from build123d import *

# Parameters (mm, degrees)
BOSS_EXTRUDE1_DEPTH = 140
SKETCH1_5_R         = 0.75
BOSS_EXTRUDE2_DEPTH = 5
SKETCH2_R           = 0.9
SKETCH2_R_2         = 0.75
CUT_EXTRUDE1_DEPTH  = 6
SKETCH3_W           = 0.25
SKETCH3_H           = 2.7
CUT_EXTRUDE2_DEPTH  = 171.537268104
SKETCH4_W           = 13
SKETCH4_H           = 1.35
SKETCH4_W_2         = 24
SKETCH4_W_3         = 6
SKETCH4_W_4         = 7
SKETCH4_W_5         = 30
SKETCH4_W_6         = 4
CUT_EXTRUDE4_DEPTH  = 86.663575277
SKETCH6_W           = 13
SKETCH6_H           = 1.35
SKETCH6_W_2         = 24
SKETCH6_W_3         = 6
SKETCH6_W_4         = 7
SKETCH6_W_5         = 4
SKETCH6_W_6         = 20
CUT_EXTRUDE5_DEPTH  = 86.765556194
SKETCH7_W           = 20
SKETCH7_H           = 1.8
CUT_EXTRUDE6_DEPTH  = 86.663575277
SKETCH8_W           = 20
SKETCH8_H           = 1.8
CUT_EXTRUDE7_DEPTH  = 86.765556194


with BuildPart() as part:
    # Sketch1 → Boss-Extrude1 (new body)
    with BuildSketch(Plane(origin=(-58.146340827, 0, 0), x_dir=(0, 0, -1), z_dir=(1, 0, 0))):
        Polygon((-20.52887033, 84.640306989), (-21.87887033, 84.640306989), (-21.87887033, 85.940306989), (-21.37887033, 85.940306989), (-21.37887033, 86.490306989), (-23.17887033, 86.490306989), (-23.17887033, 85.940306989), (-22.67887033, 85.940306989), (-22.67887033, 84.640306989), (-24.02887033, 84.640306989), (-24.02887033, 76.840306989), (-13.52887033, 76.840306989), (-13.52887033, 77.640306989), (-14.87887033, 77.640306989), (-14.87887033, 78.940306989), (-14.37887033, 78.940306989), (-14.37887033, 79.490306989), (-16.17887033, 79.490306989), (-16.17887033, 78.940306989), (-15.67887033, 78.940306989), (-15.67887033, 77.640306989), (-17.02887033, 77.640306989), (-17.02887033, 80.340306989), (-20.52887033, 80.340306989), align=None)
    extrude(amount=BOSS_EXTRUDE1_DEPTH)

    # Sketch1_5 → Boss-Extrude2 (add)
    with BuildSketch(Plane(origin=(-58.146340827, 0, 0), x_dir=(0, 0, -1), z_dir=(1, 0, 0))):
        with Locations((-22.27887033, 82.090306989)):
            Circle(SKETCH1_5_R)
        with Locations((-18.77887033, 78.590306989)):
            Circle(SKETCH1_5_R)
    extrude(amount=-BOSS_EXTRUDE2_DEPTH)

    # Sketch2 → Cut-Extrude1 (cut)
    with BuildSketch(Plane(origin=(81.853659173, 0, 0), x_dir=(0, 0, -1), z_dir=(1, 0, 0))):
        with Locations((-22.27887033, 82.090306989)):
            Circle(SKETCH2_R)
        with Locations((-22.27887033, 82.090306989)):
            Circle(SKETCH2_R_2, mode=Mode.SUBTRACT)
        with Locations((-22.27887033, 82.090306989)):
            Circle(SKETCH2_R_2)
        with Locations((-18.77887033, 78.590306989)):
            Circle(SKETCH2_R)
        with Locations((-18.77887033, 78.590306989)):
            Circle(SKETCH2_R_2, mode=Mode.SUBTRACT)
        with Locations((-18.77887033, 78.590306989)):
            Circle(SKETCH2_R_2)
    extrude(amount=-CUT_EXTRUDE1_DEPTH, mode=Mode.SUBTRACT)

    # Sketch3 → Cut-Extrude2 (cut, through all)
    with BuildSketch(Plane(origin=(81.853659173, 0, 0), x_dir=(0, 0, -1), z_dir=(1, 0, 0))):
        with Locations((-17.15387033, 78.990306989)):
            Rectangle(SKETCH3_W, SKETCH3_H)
    extrude(amount=-CUT_EXTRUDE2_DEPTH, mode=Mode.SUBTRACT)

    # Sketch4 → Cut-Extrude4 (cut, through all)
    with BuildSketch(Plane(origin=(0, 84.640306989, 0), x_dir=(1, 0, 0), z_dir=(0, 1, 0))):
        with Locations((75.353659173, -23.35387033)):
            Rectangle(SKETCH4_W, SKETCH4_H)
        with Locations((53.853659173, -21.20387033)):
            Rectangle(SKETCH4_W_2, SKETCH4_H)
        with Locations((53.853659173, -23.35387033)):
            Rectangle(SKETCH4_W_2, SKETCH4_H)
        with Locations((38.853659173, -21.20387033)):
            Rectangle(SKETCH4_W_3, SKETCH4_H)
        with Locations((38.853659173, -23.35387033)):
            Rectangle(SKETCH4_W_3, SKETCH4_H)
        with Locations((32.353659173, -21.20387033)):
            Rectangle(SKETCH4_W_4, SKETCH4_H)
        with Locations((32.353659173, -23.35387033)):
            Rectangle(SKETCH4_W_4, SKETCH4_H)
        with Locations((13.853659173, -23.35387033)):
            Rectangle(SKETCH4_W_2, SKETCH4_H)
        with Locations((13.853659173, -21.20387033)):
            Rectangle(SKETCH4_W_2, SKETCH4_H)
        with Locations((-1.146340827, -21.20387033)):
            Rectangle(SKETCH4_W_3, SKETCH4_H)
        with Locations((-1.146340827, -23.35387033)):
            Rectangle(SKETCH4_W_3, SKETCH4_H)
        with Locations((-7.646340827, -21.20387033)):
            Rectangle(SKETCH4_W_4, SKETCH4_H)
        with Locations((-7.646340827, -23.35387033)):
            Rectangle(SKETCH4_W_4, SKETCH4_H)
        with Locations((-26.146340827, -21.20387033)):
            Rectangle(SKETCH4_W_2, SKETCH4_H)
        with Locations((-26.146340827, -23.35387033)):
            Rectangle(SKETCH4_W_2, SKETCH4_H)
        with Locations((-41.146340827, -23.35387033)):
            Rectangle(SKETCH4_W_3, SKETCH4_H)
        with Locations((-41.146340827, -21.20387033)):
            Rectangle(SKETCH4_W_3, SKETCH4_H)
        with Locations((-47.646340827, -21.20387033)):
            Rectangle(SKETCH4_W_4, SKETCH4_H)
        with Locations((-47.646340827, -23.35387033)):
            Rectangle(SKETCH4_W_4, SKETCH4_H)
        with Locations((-69.146340827, -21.20387033)):
            Rectangle(SKETCH4_W_5, SKETCH4_H)
        with Locations((-56.146340827, -23.35387033)):
            Rectangle(SKETCH4_W_6, SKETCH4_H)
        with Locations((75.353659173, -21.20387033)):
            Rectangle(SKETCH4_W, SKETCH4_H)
    extrude(amount=CUT_EXTRUDE4_DEPTH, mode=Mode.SUBTRACT)

    # Sketch6 → Cut-Extrude5 (cut, through all)
    with BuildSketch(Plane(origin=(0, 77.640306989, 0), x_dir=(1, 0, 0), z_dir=(0, 1, 0))):
        with Locations((75.353659173, -16.35387033)):
            Rectangle(SKETCH6_W, SKETCH6_H)
        with Locations((75.353659173, -14.20387033)):
            Rectangle(SKETCH6_W, SKETCH6_H)
        with Locations((53.853659173, -14.20387033)):
            Rectangle(SKETCH6_W_2, SKETCH6_H)
        with Locations((53.853659173, -16.35387033)):
            Rectangle(SKETCH6_W_2, SKETCH6_H)
        with Locations((38.853659173, -14.20387033)):
            Rectangle(SKETCH6_W_3, SKETCH6_H)
        with Locations((38.853659173, -16.35387033)):
            Rectangle(SKETCH6_W_3, SKETCH6_H)
        with Locations((32.353659173, -16.35387033)):
            Rectangle(SKETCH6_W_4, SKETCH6_H)
        with Locations((32.353659173, -14.20387033)):
            Rectangle(SKETCH6_W_4, SKETCH6_H)
        with Locations((13.853659173, -16.35387033)):
            Rectangle(SKETCH6_W_2, SKETCH6_H)
        with Locations((13.853659173, -14.20387033)):
            Rectangle(SKETCH6_W_2, SKETCH6_H)
        with Locations((-1.146340827, -16.35387033)):
            Rectangle(SKETCH6_W_3, SKETCH6_H)
        with Locations((-1.146340827, -14.20387033)):
            Rectangle(SKETCH6_W_3, SKETCH6_H)
        with Locations((-7.646340827, -14.20387033)):
            Rectangle(SKETCH6_W_4, SKETCH6_H)
        with Locations((-7.646340827, -16.35387033)):
            Rectangle(SKETCH6_W_4, SKETCH6_H)
        with Locations((-26.146340827, -14.20387033)):
            Rectangle(SKETCH6_W_2, SKETCH6_H)
        with Locations((-26.146340827, -16.35387033)):
            Rectangle(SKETCH6_W_2, SKETCH6_H)
        with Locations((-41.146340827, -14.20387033)):
            Rectangle(SKETCH6_W_3, SKETCH6_H)
        with Locations((-41.146340827, -16.35387033)):
            Rectangle(SKETCH6_W_3, SKETCH6_H)
        with Locations((-47.646340827, -16.35387033)):
            Rectangle(SKETCH6_W_4, SKETCH6_H)
        with Locations((-47.646340827, -14.20387033)):
            Rectangle(SKETCH6_W_4, SKETCH6_H)
        with Locations((-56.146340827, -14.20387033)):
            Rectangle(SKETCH6_W_5, SKETCH6_H)
        with Locations((-66.146340827, -16.35387033)):
            Rectangle(SKETCH6_W_2, SKETCH6_H)
        with Locations((-68.146340827, -14.20387033)):
            Rectangle(SKETCH6_W_6, SKETCH6_H)
    extrude(amount=CUT_EXTRUDE5_DEPTH, mode=Mode.SUBTRACT)

    # Sketch7 → Cut-Extrude6 (cut, through all)
    with BuildSketch(Plane(origin=(0, 84.640306989, 0), x_dir=(1, 0, 0), z_dir=(0, 1, 0))):
        with Locations((55.853659173, -22.27887033)):
            Rectangle(SKETCH7_W, SKETCH7_H)
        with Locations((15.853659173, -22.27887033)):
            Rectangle(SKETCH7_W, SKETCH7_H)
        with Locations((-24.146340827, -22.27887033)):
            Rectangle(SKETCH7_W, SKETCH7_H)
        with Locations((-64.146340827, -22.27887033)):
            Rectangle(SKETCH7_W, SKETCH7_H)
    extrude(amount=CUT_EXTRUDE6_DEPTH, mode=Mode.SUBTRACT)

    # Sketch8 → Cut-Extrude7 (cut, through all)
    with BuildSketch(Plane(origin=(0, 77.640306989, 0), x_dir=(1, 0, 0), z_dir=(0, 1, 0))):
        with Locations((55.853659173, -15.27887033)):
            Rectangle(SKETCH8_W, SKETCH8_H)
        with Locations((15.853659173, -15.27887033)):
            Rectangle(SKETCH8_W, SKETCH8_H)
        with Locations((-24.146340827, -15.27887033)):
            Rectangle(SKETCH8_W, SKETCH8_H)
        with Locations((-64.146340827, -15.27887033)):
            Rectangle(SKETCH8_W, SKETCH8_H)
    extrude(amount=CUT_EXTRUDE7_DEPTH, mode=Mode.SUBTRACT)


solid = part.part
Input: part model. Units: mm. Frame: model coordinates. A direction names the side the tool comes from. Coordinates: 2 decimals unless noted, no trailing zeros. Loops run counter-clockwise (first coordinate to the right, second up) from the corner with the lowest first, then second, coordinate; pieces in that order, holes last.
(1) Pull-direction query (Z, two-part tool) for faces 4 (the face through (11, 76.84, 19)), 5 (the face through (11, 82, 20.529)), 6 (the face through (13, 77.64, 15)); classes: released by +Z, released by -Z, zero draft, split by the parting line, or undercut.
(2) Material intervals for probe 1 along Z at (x, y) = (-47, 79.25); probe 2 along Y at (x, z) = (-55, 18.75); probe 3 along X at (y, z) = (83, 21.25), sorted ascending.
(3) Section B-B on x = 32. Return the cut outline in (y, z), then the cut area to 3 significant figures.
(4) Set-up query: faces 1 (the face through (11, 81, 24.029)), 2 (the face through (11, 80.34, 19)), 3 (the face through (13, 79, 17.279)). Return all of +Z, -Z, +X, -X, +Y, -Y with unobstructed straight access to the full face (end or side cutting, diameter ignored); none if empty.
(5) Section A-A on x = -26. Return the cut outline in (y, z).
(6) First-contact query: pin 1 Ø0.6 at (x, y) = (27, 86.5) entering from -Z; pin 2 Ø0.6 at (x, y) = (-53.5, 79) entering from -Z; pin 3 Ø1.5 at (x, y) = (37.5, 86) entering from -Z. Flat tips, straight axial feed; report the tip coordinate or a pass-through.
Data:
1. face 4: zero draft
1. face 5: released by -Z
1. face 6: undercut
2. probe 1: z = 14.88 to 15.68, 17.28 to 24.03
2. probe 2: y = 76.84 to 80.34
2. probe 3: x = -58.15 to 81.85
3. outline: (76.84, 13.53) - (77.64, 13.53) - (77.64, 14.88) - (79.49, 14.88) - (79.49, 15.68) - (77.64, 15.68) - (77.64, 17.28) - (80.34, 17.28) - (80.34, 20.53) - (84.64, 20.53) - (84.64, 21.88) - (86.49, 21.88) - (86.49, 22.68) - (84.64, 22.68) - (84.64, 24.03) - (76.84, 24.03) - close
3. area: 44.6 mm2
4. face 1: +Z, +X, -X, +Y, -Y
4. face 2: -Z, +X, -X, +Y
4. face 3: +X, -X, +Y
5. outline: (76.84, 13.53) - (77.64, 13.53) - (77.64, 17.28) - (80.34, 17.28) - (80.34, 20.53) - (84.64, 20.53) - (84.64, 24.03) - (76.84, 24.03) - close
6. pin 1: stops at z = 21.38
6. pin 2: stops at z = 14.38
6. pin 3: stops at z = 21.88
